```python
from build123d import *

# Parameters (mm, degrees)
F0_R     = 2
F1_DEPTH = 1.4
F2_R     = 1


with BuildPart() as f1:
    # F0 (on Right) → F1 (new body)
    with BuildSketch(Plane.YZ):
        Polygon((-35.25, -14.9), (-9.2, -14.9), (-9.2, -13.4), (-9.2, -11.2), (-7.5, -11.2), (-7.5, -13.4), (8.7, -13.4), (8.7, -11.1), (12.75, -11.1), (12.75, -4), (14.15, -4), (14.15, -11.1), (18.2, -11.1), (18.2, -13.4), (38.5, -13.4), (38.5, -11.1), (42.35, -11.1), (42.35, 5.8), (43.75, 5.8), (43.75, 1.1), (49.9, 1.1), (49.9, 14.9), (-49.9, 14.9), (-49.9, 6.4402827993), (-49.9, 2.1), (-49.9, -0.1), (-43.65, -0.1), (-43.65, 2.1), (-42.25, 2.1), (-42.25, -11.1), (-39.75, -11.1), (-39.75, -13.4), (-36.95, -13.4), (-36.95, -11.2), (-35.25, -11.2), (-35.25, -13.4), align=None)
        with Locations((-22.225, -7.9)):
            Circle(F0_R, mode=Mode.SUBTRACT)
        with Locations((28.35, -7.9)):
            Circle(F0_R, mode=Mode.SUBTRACT)
        with Locations((-22.225, 7.9)):
            Circle(F0_R, mode=Mode.SUBTRACT)
        with Locations((28.35, 7.9)):
            Circle(F0_R, mode=Mode.SUBTRACT)
    extrude(amount=F1_DEPTH)

    # F2
    f2_edges = [f1.edges().sort_by_distance(p)[0] for p in [
        (0.7, -49.9, 14.9),
        (0.7, 49.9, 14.9),
        (0.7, 49.9, 1.1),
    ]]
    fillet(f2_edges, radius=F2_R)


solid = f1.part
```
Read the model definition and answer for the solid it produces. Units are mm, in the model's axes. Coordinates: 2 decimals unless noted, no trailing zeros. Write each loop counter-clockwise with the first axis right and the second up, starting at its lowest first coordinate (ties: lowest second). Pieces come first, ordered by that corner, then holes. Notation, with made-up numbers: (-27.5, -12.75) - (-2.5, -12.75) arc R7 cw to (-2.5, -1.75) - close; hole circle Ø8 at (54, -36.5). An arc over 180 degrees is marked (long way). Answer as a JSON object with one key per item and string values. Group by question number.
1. A cutting plane is placed at D-D (x = 0.95). Give the number of separate pieces and of enclosed holes in the cut face, plus the area to 3 significant figures.
2. The mould has two halves that part along Y. Classify faces 1 (the flat face through (0, -1, 0)), 2 (the cylindrical face through (0.69, -20.317, 8.501)): +Y half, -Y half, draft (parallel to the pull), parting line (faces both ways), or undercut.
3. Each of these flat-tipped pins is pushed along its axis until it touches: P1, Ø0.7, axis at x = 1, y = 32, coming from the -Z side; P2, Ø0.7, axis at x = 1, z = -12, coming from the +Y side. Where does it stop, or does it pass through?
4. A cutting plane is placed at B-B (y = 28.35). Determine the outline of the cut face in (x, z), plus the area to 3 significant figures.
5. A cutting plane is placed at A-A (z = -7.9). Determine the outline of the cut face in (x, y) (3 decimals).
6. A cutting plane is placed at C-C (z = 7.9). Determine the outline of the cut face in (x, y) (3 decimals), plus the area to 3 significant figures.
7. Consider L1, parallel to Z at x = 0.85, y = 28.35; L2, parallel to Y at x = 0.55, z = 0; L3, parallel to Y at x = 1.1, z = 3. Determine where each line is inside the solid, lowest interval first. Write a range as [from, to].
Worked out:
{
 "1": {"separate pieces": "1", "enclosed holes": "4", "area": "2,540 mm²"},
 "2": {"face 1": "draft", "face 2": "undercut"},
 "3": {"P1": "stops at z = -13.4", "P2": "stops at y = 38.5"},
 "4": {"outline": "(0, -13.4) - (1.4, -13.4) - (1.4, -9.9) - (0, -9.9) - close; (0, -5.9) - (1.4, -5.9) - (1.4, 5.9) - (0, 5.9) - close; (0, 9.9) - (1.4, 9.9) - (1.4, 14.9) - (0, 14.9) - close", "area": "28.4 mm²"},
 "5": {"outline": "(0, -42.25) - (1.4, -42.25) - (1.4, -24.225) - (0, -24.225) - close; (0, -20.225) - (1.4, -20.225) - (1.4, 12.75) - (0, 12.75) - close; (0, 14.15) - (1.4, 14.15) - (1.4, 26.35) - (0, 26.35) - close; (0, 30.35) - (1.4, 30.35) - (1.4, 42.35) - (0, 42.35) - close"},
 "6": {"outline": "(0, -49.9) - (1.4, -49.9) - (1.4, -24.225) - (0, -24.225) - close; (0, -20.225) - (1.4, -20.225) - (1.4, 26.35) - (0, 26.35) - close; (0, 30.35) - (1.4, 30.35) - (1.4, 49.9) - (0, 49.9) - close", "area": "129 mm²"},
 "7": {"L1": "z = [-13.4, -9.9], [-5.9, 5.9], [9.9, 14.9]", "L2": "y = [-49.9, -43.65], [-42.25, 42.35]", "L3": "y = [-49.9, 42.35], [43.75, 49.9]"}
}
